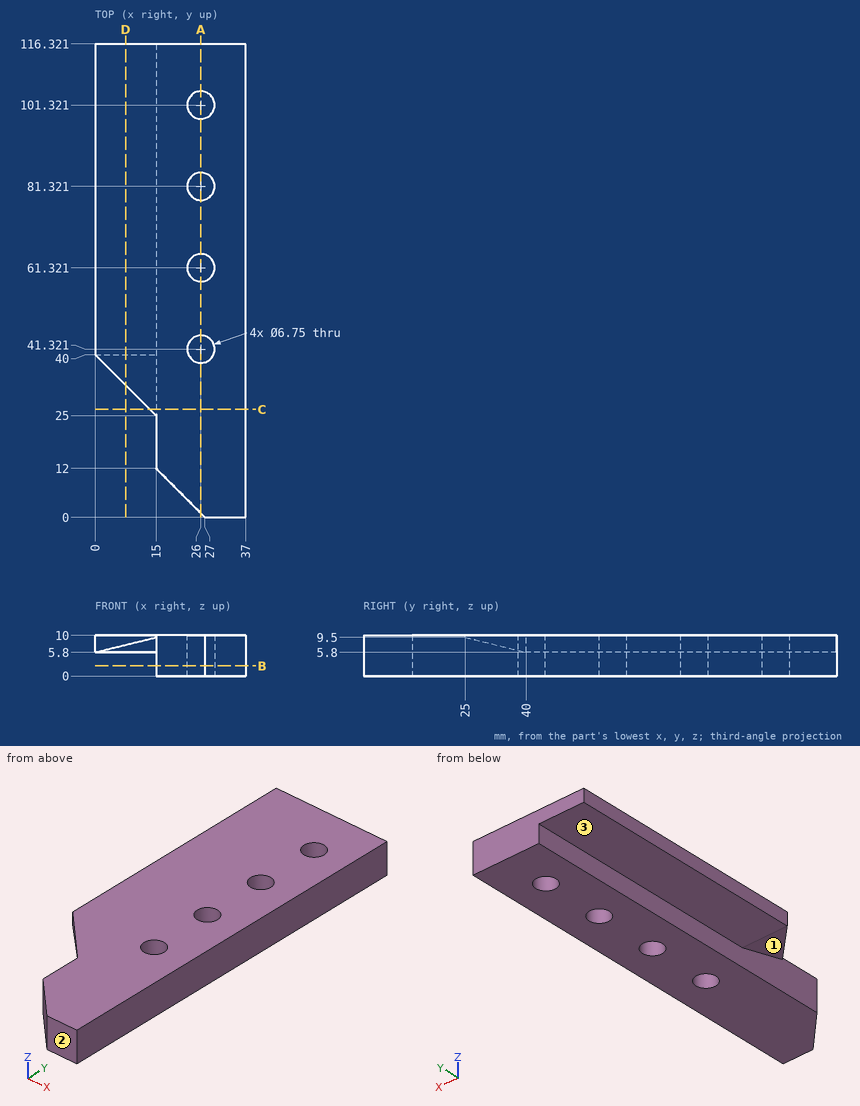
Check sheet for the drawn part. Datum: minimum x, y, z corner. Units: mm. A direction names the side the tool comes from. Give positions to 0.01 mm unless a question says otherwise; leave off trailing zeros. Loops run counter-clockwise (first coordinate to the right, second up) from the corner with the lowest first, then second, coordinate; pieces in that order, holes last. Notation, with made-up numbers: M 52,-28 L 69,-28 A25 cw 69,-2 Z; hole C 0.5,46.25 d4. An arc over 180 degrees is marked long. Return JSON: item names as keys, results as strings.
1) Gauge pin test, flat end, axial feed: P1, Ø4, axis at x = 5, y = 60.5, coming from the -Z side. Record the tip position at first contact, or that the pin passes through.
Findings:
{"P1": "stops at z = 5.8"}
2) Section check D-D, the plane x = 7.5. Enter the section's corners in (y, z).
Findings:
{"outline": "M 32.5,7.65 L 40,5.8 L 116.32,5.8 L 116.32,10 L 32.5,10 Z"}
3) Section check B-B, the plane z = 2.5. Enter the section's corners in (x, y) (3 decimals).
Findings:
{"outline": "M 15,12 L 27,0 L 37,0 L 37,116.321 L 15,116.321 Z; hole C 26,41.321 d6.75; hole C 26,61.321 d6.75; hole C 26,81.321 d6.75; hole C 26,101.321 d6.75"}
4) Section check C-C, the plane y = 26.5. Enter the section's corners in (x, z).
Findings:
{"outline": "M 13.5,9.13 L 15,9.13 L 15,0 L 37,0 L 37,10 L 13.5,10 Z"}
5) Section check A-A, the plane x = 26. Enter the section's corners in (y, z).
Findings:
{"outline": "M 1,0 L 37.95,0 L 37.95,10 L 1,10 Z; M 44.7,0 L 57.95,0 L 57.95,10 L 44.7,10 Z; M 64.7,0 L 77.95,0 L 77.95,10 L 64.7,10 Z; M 84.7,0 L 97.95,0 L 97.95,10 L 84.7,10 Z; M 104.7,0 L 116.32,0 L 116.32,10 L 104.7,10 Z"}
6) Tool access check on the marked faces 1, 2 and 3. Record the directions out of +Z, -Z, +X, -X, +Y, -Y that give a thin tool (end or side, any length) a straight path to the whole face; none if there is none.
Findings:
{"face 1": "-Z, -X, -Y", "face 2": "+Z, -Z, +X, -X, -Y", "face 3": "-Z, -X, +Y, -Y"}
7) Material ranges on L1, parallel to Y at x = 26, z = 4.75; L2, parallel to X at y = 41, z = 6.75; L3, parallel to X at y = 25, z = 2.5, recorded low to high. Write a range as [from, to].
Findings:
{"L1": "y = [1, 37.95], [44.7, 57.95], [64.7, 77.95], [84.7, 97.95], [104.7, 116.32]", "L2": "x = [0, 22.64], [29.36, 37]", "L3": "x = [15, 37]"}
